Input: dimensioned drawing with shaded views. Units: mm. Origin: part minimum x, y, z. Round coordinates to 2 decimals unless told otherwise and drop trailing zeros. Loops run counter-clockwise (first coordinate to the right, second up) from the corner with the lowest first, then second, coordinate; pieces in that order, holes last. Notation, with made-up numbers: (50, 71) - (71, 71) arc R15 cw to (71, 95) - close; hole circle Ø9 at (70.5, 59). An arc over 180 degrees is marked (long way). One line per question, with ' | ' between items.
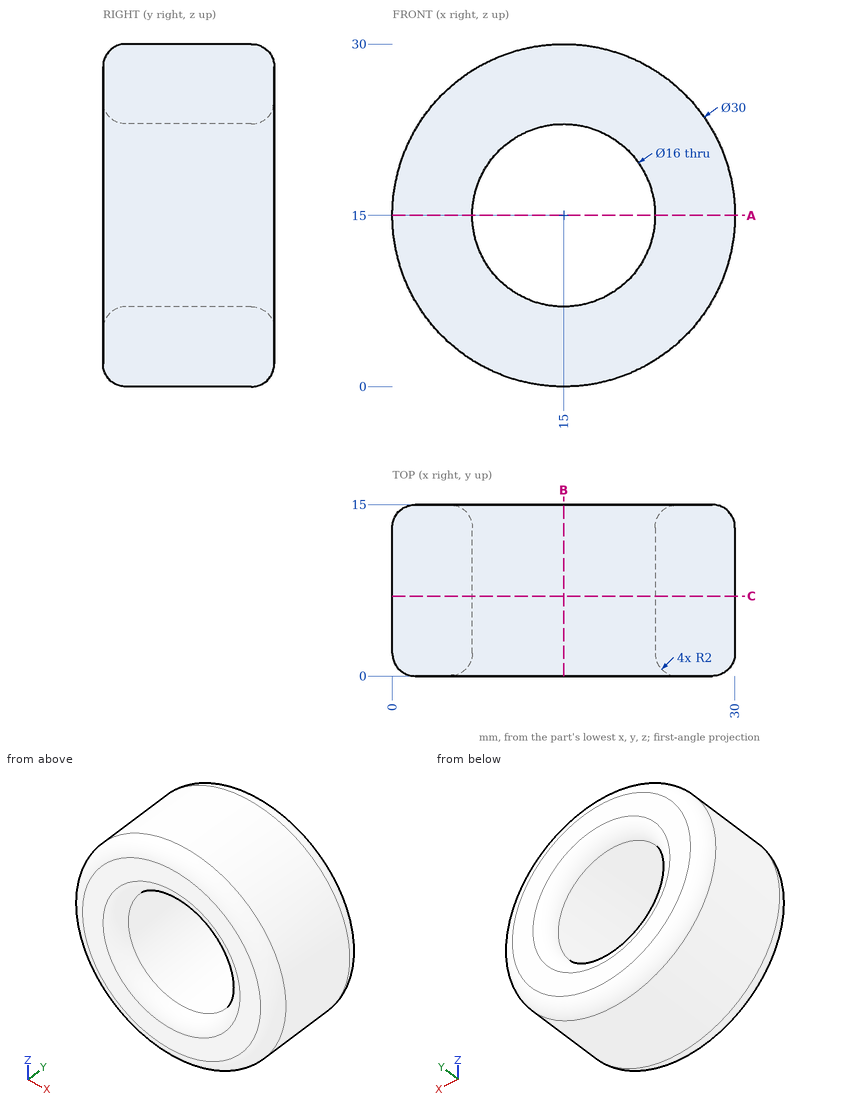
1. Material intervals for probe 1 along Z at (x, y) = (15, 5.5); probe 2 along Z at (x, y) = (8.25, 11.5); probe 3 along X at (y, z) = (5.5, 20) (3 decimals), sorted ascending.
Worked out:
probe 1: z = 0 to 7, 23 to 30 | probe 2: z = 1.6 to 10.71, 19.29 to 28.4 | probe 3: x = 0.858 to 8.755, 21.245 to 29.142
2. Contact query for flat-ended pins moving along their axis: P1, Ø8, axis at y = 10.5, z = 26.5, coming from the +X side; P2, Ø1.5, axis at x = 26.5, y = 11, coming from the +Z side; P3, Ø2, axis at y = 2.5, z = 10, coming from the +X side. Output: stop coordinate, or through.
Worked out:
P1: stops at x = 27.99 | P2: stops at z = 25.46 | P3: stops at x = 29.46
3. Section query B-B, the plane x = 15. Return loops of the section in (y, z).
Worked out:
outline: (0, 2) arc R2 ccw to (2, 0) - (13, 0) arc R2 ccw to (15, 2) - (15, 5) arc R2 ccw to (13, 7) - (2, 7) arc R2 ccw to (0, 5) - close; (0, 25) arc R2 ccw to (2, 23) - (13, 23) arc R2 ccw to (15, 25) - (15, 28) arc R2 ccw to (13, 30) - (2, 30) arc R2 ccw to (0, 28) - close
4. Section query C-C, the plane y = 7. Return loops of the section in (x, z).
Worked out:
outline: circle Ø30 at (15, 15); hole circle Ø16 at (15, 15)
5. Section query A-A, the plane z = 15. Return loops of the section in (x, y), plus the area to 3 significant figures.
Worked out:
outline: (0, 2) arc R2 ccw to (2, 0) - (5, 0) arc R2 ccw to (7, 2) - (7, 13) arc R2 ccw to (5, 15) - (2, 15) arc R2 ccw to (0, 13) - close; (23, 2) arc R2 ccw to (25, 0) - (28, 0) arc R2 ccw to (30, 2) - (30, 13) arc R2 ccw to (28, 15) - (25, 15) arc R2 ccw to (23, 13) - close | area: 203 mm2
